Build history of the part. All positions in model axes, mm. Coordinates: 2 decimals unless noted, no trailing zeros. Loops run counter-clockwise (first coordinate to the right, second up) from the corner with the lowest first, then second, coordinate; pieces in that order, holes last.
Item 1: Cut at A-A (x = -5). List the corners of the cut face in (y, z).
Item 2: Cut at D-D (y = -9.5). List the corners of the cut face in (x, z).
Item 3: Cut at C-C (z = -35). List the corners of the cut face in (x, y), and give its area (3 significant figures).
Item 4: Cut at B-B (y = -7). List the corners of the cut face in (x, z), and give its area (3 significant figures).
Item 5: Drill centre lines: line 1 along X through (y, z) = (-5, -35); line 2 along Z through (x, y) = (-5.5, -1.5); line 3 along Z through (x, y) = (-4, -6.5). Where is each one in solid material? Low to high.
from build123d import *

# Parameters (mm, degrees)
SKIZZE1_W                       = 10
SKIZZE1_H                       = 40
SKIZZE1_R                       = 1.75
AUFSATZ_LINEAR_AUSTRAGEN1_DEPTH = 10
VERRUNDUNG1_R                   = 1


with BuildPart() as part:
    # Skizze1 → Aufsatz-Linear austragen1 (new body)
    with BuildSketch(Plane(origin=(0, 0, 0), x_dir=(1, 0, 0), z_dir=(0, 1, 0))):
        with Locations((-5, 20)):
            Rectangle(SKIZZE1_W, SKIZZE1_H)
        with Locations(Location((-5, 35, 0), (0, 0, 270))):
            Circle(SKIZZE1_R, mode=Mode.SUBTRACT)
    extrude(amount=-AUFSATZ_LINEAR_AUSTRAGEN1_DEPTH)

    # Verrundung1
    verrundung1_edges = [part.edges().sort_by_distance(p)[0] for p in [
        (-5, 0, -40),
        (-5, -10, -40),
        (-10, -5, -40),
        (0, -5, -40),
    ]]
    fillet(verrundung1_edges, radius=VERRUNDUNG1_R)


solid = part.part
Filled sheet:
1. outline: (-10, -39) arc R1 ccw to (-9, -40) - (-1, -40) arc R1 ccw to (0, -39) - (0, -36.75) - (-10, -36.75) - close; (-10, -33.25) - (0, -33.25) - (0, 0) - (-10, 0) - close
2. outline: (-10, -39) arc R1 ccw to (-9.5, -39.87) - (-0.5, -39.87) arc R1 ccw to (0, -39) - (0, 0) - (-10, 0) - close; hole circle Ø3.5 at (-5, -35)
3. outline: (-10, -10) - (-6.75, -10) - (-6.75, 0) - (-10, 0) - close; (-3.25, -10) - (0, -10) - (0, 0) - (-3.25, 0) - close
3. area: 65.0 mm2
4. outline: (-10, -39) arc R1 ccw to (-9, -40) - (-1, -40) arc R1 ccw to (0, -39) - (0, 0) - (-10, 0) - close; hole circle Ø3.5 at (-5, -35)
4. area: 390 mm2
5. line 1: x = -10 to -6.75, -3.25 to 0
5. line 2: z = -40 to -36.68, -33.32 to 0
5. line 3: z = -40 to -36.44, -33.56 to 0
